Input: part model. Units: mm. Frame: model coordinates. Give positions to 0.01 mm unless a question says otherwise; leave off trailing zeros. Order: outer loops, then holes, each group sorted by start corner. A loop starts at its lowest first (then second) coordinate and runs counter-clockwise, first axis right, second up. Notation, with made-up numbers: (-16, 35) - (17, 35) arc R27 cw to (17, 70) - close; hole circle Ø5 at (-36.75, 13). An arc over 180 degrees is marked (long way). Use a Markdown table: item, result.
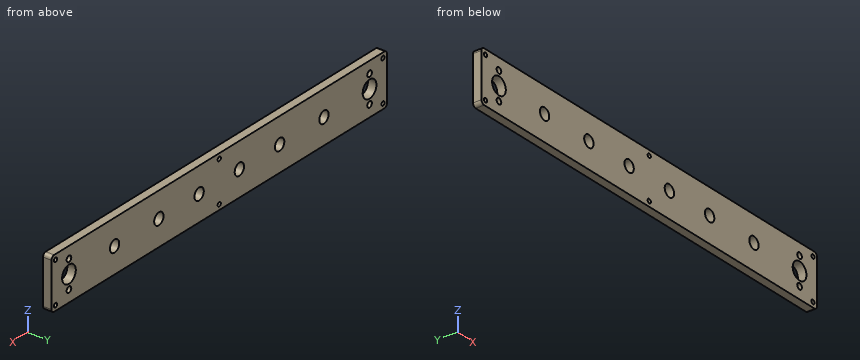
from build123d import *

# Parameters (mm, degrees)
SKETCH1_W           = 317.5
SKETCH1_H           = 38.1
BOSS_EXTRUDE1_DEPTH = 3.175
SKETCH2_R           = 4.4196
SKETCH2_R_2         = 6.477
SKETCH2_R_3         = 2.19075
CUT_EXTRUDE1_DEPTH  = 161.014960238
SKETCH3_R           = 1.5113
CUT_EXTRUDE2_DEPTH  = 161.014960238
FILLET1_R           = 2.54


with BuildPart() as part:
    # Sketch1 → Boss-Extrude1 (new, symmetric)
    with BuildSketch(Plane(origin=(0, 0, 0), x_dir=(1, 0, 0), z_dir=(0, 1, 0))):
        Rectangle(SKETCH1_W, SKETCH1_H)
    extrude(amount=BOSS_EXTRUDE1_DEPTH, both=True)

    # Sketch2 → Cut-Extrude1 (cut, through all)
    with BuildSketch(Plane(origin=(0, 3.175, 0), x_dir=(1, 0, 0), z_dir=(0, 1, 0))):
        with Locations(Location((-99.06, 0, 0), (0, 0, 270))):
            Circle(SKETCH2_R)
        with Locations(Location((-57.15, 0, 0), (0, 0, 270))):
            Circle(SKETCH2_R)
        with Locations(Location((-19.05, 0, 0), (0, 0, 270))):
            Circle(SKETCH2_R)
        with Locations(Location((19.05, 0, 0), (0, 0, 270))):
            Circle(SKETCH2_R)
        with Locations(Location((57.15, 0, 0), (0, 0, 270))):
            Circle(SKETCH2_R)
        with Locations(Location((-142.24, 0, 0), (0, 0, 270))):
            Circle(SKETCH2_R_2)
        with Locations(Location((-142.24, -10.31875, 0), (0, 0, 270))):
            Circle(SKETCH2_R_3)
        with Locations(Location((-142.24, 10.31875, 0), (0, 0, 270))):
            Circle(SKETCH2_R_3)
        with Locations(Location((142.24, 0, 0), (0, 0, 270))):
            Circle(SKETCH2_R_2)
        with Locations(Location((142.24, -10.31875, 0), (0, 0, 270))):
            Circle(SKETCH2_R_3)
        with Locations(Location((142.24, 10.31875, 0), (0, 0, 270))):
            Circle(SKETCH2_R_3)
        with Locations(Location((99.06, 0, 0), (0, 0, 270))):
            Circle(SKETCH2_R)
    extrude(amount=-CUT_EXTRUDE1_DEPTH, mode=Mode.SUBTRACT)

    # Sketch3 → Cut-Extrude2 (cut, through all)
    with BuildSketch(Plane(origin=(0, 3.175, 0), x_dir=(1, 0, 0), z_dir=(0, 1, 0))):
        with Locations(Location((-154.94, 15.24, 0), (0, 0, 270))):
            Circle(SKETCH3_R)
        with Locations(Location((-154.94, -15.24, 0), (0, 0, 270))):
            Circle(SKETCH3_R)
        with Locations(Location((154.94, -15.24, 0), (0, 0, 270))):
            Circle(SKETCH3_R)
        with Locations(Location((154.94, 15.24, 0), (0, 0, 270))):
            Circle(SKETCH3_R)
        with Locations(Location((0, 15.24, 0), (0, 0, 270))):
            Circle(SKETCH3_R)
        with Locations(Location((0, -15.24, 0), (0, 0, 270))):
            Circle(SKETCH3_R)
    extrude(amount=-CUT_EXTRUDE2_DEPTH, mode=Mode.SUBTRACT)

    # Fillet1
    fillet1_edges = [part.edges().sort_by_distance(p)[0] for p in [
        (158.75, 0, 19.05),
        (-158.75, 0, 19.05),
        (-158.75, 0, -19.05),
        (158.75, 0, -19.05),
    ]]
    fillet(fillet1_edges, radius=FILLET1_R)


solid = part.part
1. Section query B-B (y = 0.75). State how many separate pieces and enclosed holes the cut face has, then the cut area to 3 significant figures.
Response:
| item | result |
|---|---|
| separate pieces | 1 |
| enclosed holes | 18 |
| area | 11,400 mm^2 |
2. Pin query (flat end, axial travel): pin 1 (14 mm diameter, centred on x = -57.15, z = 0, fed in from -Y) (3 decimals). Return the tip coordinate at first contact, or that it passes through.
Response:
| item | result |
|---|---|
| pin 1 | stops at y = -3.175 |
3. Material intervals for line 1 along Z through (x, y) = (154.94, 1.75); line 2 along X through (y, z) = (2.5, 5.5); line 3 along X through (y, z) = (-2, -9.5), sorted ascending.
Response:
| item | result |
|---|---|
| line 1 | z = -19.05 to -16.75, -13.73 to 13.73, 16.75 to 19.05 |
| line 2 | x = -158.75 to -145.66, -138.82 to 138.82, 145.66 to 158.75 |
| line 3 | x = -158.75 to -144.27, -140.21 to 140.21, 144.27 to 158.75 |
4. Section query A-A (x = 99.06). Return loops of the section in (y, z) (3 decimals), then the cut area to 3 significant figures.
Response:
| item | result |
|---|---|
| outline | (-3.175, -19.05) - (3.175, -19.05) - (3.175, -4.42) - (-3.175, -4.42) - close; (-3.175, 4.42) - (3.175, 4.42) - (3.175, 19.05) - (-3.175, 19.05) - close |
| area | 186 mm^2 |
